Design review of the part built by this model. Coordinates are the model's own, in mm. Face numbers are marked on the shaded views. A direction names the side the tool comes from. Coordinates: 2 decimals unless noted, no trailing zeros. Write each loop counter-clockwise with the first axis right and the second up, starting at its lowest first coordinate (ties: lowest second). Pieces come first, ordered by that corner, then holes.
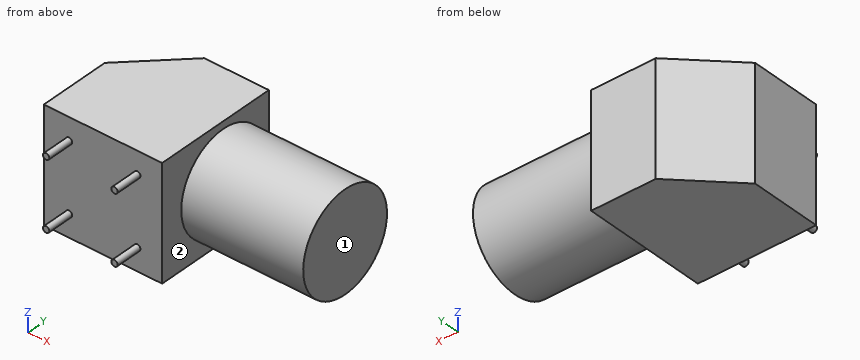
```python
from build123d import *

# Parameters (mm, degrees)
ESQUISSE1_W      = 13.2
ESQUISSE1_H      = 12.6
EXTRUSION1_DEPTH = 14
CHANFREIN1_SIZE  = 6
ESQUISSE2_R      = 5.5
EXTRUSION2_DEPTH = 13.6
ESQUISSE3_R      = 0.35
EXTRUSION3_DEPTH = 3


with BuildPart() as part:
    # Esquisse1 → Extrusion1 (new body)
    with BuildSketch(Plane(origin=(0, 0, 0), x_dir=(1, 0, 0), z_dir=(0, 1, 0))):
        with Locations((6.6, 6.3)):
            Rectangle(ESQUISSE1_W, ESQUISSE1_H)
    extrude(amount=EXTRUSION1_DEPTH)

    # Chanfrein1
    chanfrein1_edges = [part.edges().sort_by_distance(p)[0] for p in [
        (0, 14, -6.3),
    ]]
    chamfer(chanfrein1_edges, length=CHANFREIN1_SIZE)

    # Esquisse2 → Extrusion2 (add)
    with BuildSketch(Plane(origin=(13.2, 0, 0), x_dir=(0, 0, -1), z_dir=(1, 0, 0))):
        with Locations(Location((6.3, 8, 0), (0, 0, 180))):
            Circle(ESQUISSE2_R)
    extrude(amount=EXTRUSION2_DEPTH)

    # Esquisse3 → Extrusion3 (add)
    with BuildSketch(Plane.XZ):
        with Locations(Location((10.43, -2.49, 0), (0, 0, 270))):
            Circle(ESQUISSE3_R)
        with Locations(Location((10.43, -10.11, 0), (0, 0, 270))):
            Circle(ESQUISSE3_R)
        with Locations(Location((2.81, -2.49, 0), (0, 0, 270))):
            Circle(ESQUISSE3_R)
        with Locations(Location((2.81, -10.11, 0), (0, 0, 270))):
            Circle(ESQUISSE3_R)
    extrude(amount=EXTRUSION3_DEPTH)


solid = part.part
```
(1) Wall thickness on line 1 (X direction, y = 5.25, z = -11.5); line 2 (Y direction, x = 12.5, z = -9.5); line 3 (Z direction, x = 20, y = 9): over which ranges is each line inside the solid? List them lowest first.
(2) Consider section B-B (z = -6.3). Give the boundary of the cut face in (x, y), plus the area to 3 significant figures.
(3) Consider section A-A (x = 10.43). Give the boundary of the cut face in (y, z), plus the area to 3 significant figures.
(4) Insertion check: pin 1 Ø1.5 at (y, z) = (2.5, -11) entering from +X; pin 2 Ø4 at (x, z) = (5.5, -9) entering from -Y; pin 3 Ø1 at (x, z) = (22, -6.5) entering from -Y. Each pin has a flat end and moves straight along its axis. Give the tip position at first contact, or say it passes through.
(5) For the marked faces 1 and 2, list the 3-axis set-ups (+Z, -Z, +X, -X, +Y, -Y) from which the entire face can be reached by the end or side of a thin tool; tool diameter is ignored.
(6) Consider section C-C (y = -0.5). Give the boundary of the cut face in (x, z), plus the area to 3 significant figures.
(7) Consider section D-D (y = 13). Give the boundary of the cut face in (x, z), plus the area to 3 significant figures.
Results:
1. line 1: x = 0 to 13.2
1. line 2: y = 0 to 14
1. line 3: z = -11.71 to -0.89
2. outline: (0, 0) - (13.2, 0) - (13.2, 2.5) - (26.8, 2.5) - (26.8, 13.5) - (13.2, 13.5) - (13.2, 14) - (6, 14) - (0, 8) - close
2. area: 316 mm2
3. outline: (-3, -10.46) - (0, -10.46) - (0, -12.6) - (14, -12.6) - (14, 0) - (0, 0) - (0, -2.14) - (-3, -2.14) - (-3, -2.84) - (0, -2.84) - (0, -9.76) - (-3, -9.76) - close
3. area: 181 mm2
4. pin 1: stops at x = 13.2
4. pin 2: stops at y = 0
4. pin 3: stops at y = 2.5
5. face 1: +Z, -Z, +X, +Y, -Y
5. face 2: +X
6. outline: circle Ø0.7 at (2.81, -10.11); circle Ø0.7 at (2.81, -2.49); circle Ø0.7 at (10.43, -10.11); circle Ø0.7 at (10.43, -2.49)
6. area: 1.54 mm2
7. outline: (5, -12.6) - (13.2, -12.6) - (13.2, -8.59) - (26.8, -8.59) - (26.8, -4.01) - (13.2, -4.01) - (13.2, 0) - (5, 0) - close
7. area: 166 mm2
